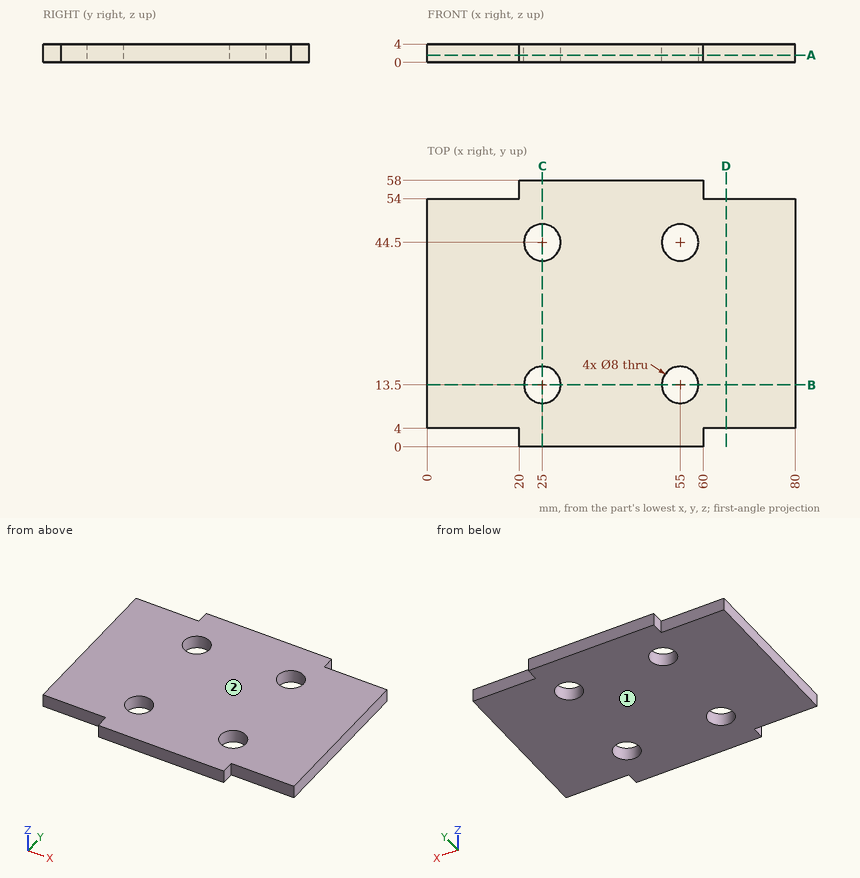
For this review, use the dimensioned drawing (mm, ordinates from the lowest corner) and the shaded views. Give positions to 0.01 mm unless a question says otherwise; leave off trailing zeros. Order: outer loops, then holes, each group sorted by start corner. A loop starts at its lowest first (then second) coordinate and runs counter-clockwise, first axis right, second up. Notation, with made-up numbers: (34, -26) - (87, -26) arc R22 cw to (87, -13) - close; hole circle Ø11 at (59.5, 64). An arc over 180 degrees is marked (long way). Use a Markdown table: item, result. Add a question column.
(1) Add section B-B on y = 13.5. Give the boundary of the cut face in (x, z), then the cut area to 3 significant figures.
(2) Add section D-D on x = 65. Give the boundary of the cut face in (y, z), then the cut area to 3 significant figures.
(3) Add section A-A on z = 1.6. Give the boundary of the cut face in (x, y), then the cut area to 3 significant figures.
(4) Mouldability with a two-part tool opening along Z and no side actions: class the marked faces 1 and 2 as +Z half, -Z half, draft (parallel to the pull), parting line (faces both ways), or undercut.
(5) Clearance check with flat-ended pins moving along their axes: P1, Ø1.2, axis at x = 66, z = 2, coming from the +Y side; P2, Ø5, axis at x = 55, y = 44.5, coming from the +Z side; P3, Ø2, axis at y = 1.5, z = 2.5, coming from the -X side. State where each tip first meets the part, or that it passes through.
(6) Add section C-C on x = 25. Give the boundary of the cut face in (y, z).
(7) Wall thickness on probe 1 along Y at (x, z) = (55, 3.2); probe 2 along X at (y, z) = (14.5, 3.5); probe 3 along Y at (x, z) = (73, 2.7): over which ranges is each line inside the solid? List them lowest first. Write a range as [from, to].
Report:
| question | item | result |
|---|---|---|
| 1 | outline | (0, 0) - (21, 0) - (21, 4) - (0, 4) - close; (29, 0) - (51, 0) - (51, 4) - (29, 4) - close; (59, 0) - (80, 0) - (80, 4) - (59, 4) - close |
| 1 | area | 256 mm² |
| 2 | outline | (4, 0) - (54, 0) - (54, 4) - (4, 4) - close |
| 2 | area | 200 mm² |
| 3 | outline | (0, 4) - (20, 4) - (20, 0) - (60, 0) - (60, 4) - (80, 4) - (80, 54) - (60, 54) - (60, 58) - (20, 58) - (20, 54) - (0, 54) - close; hole circle Ø8 at (25, 13.5); hole circle Ø8 at (25, 44.5); hole circle Ø8 at (55, 13.5); hole circle Ø8 at (55, 44.5) |
| 3 | area | 4,120 mm² |
| 4 | face 1 | -Z half |
| 4 | face 2 | +Z half |
| 5 | P1 | stops at y = 54 |
| 5 | P2 | passes through |
| 5 | P3 | stops at x = 20 |
| 6 | outline | (0, 0) - (9.5, 0) - (9.5, 4) - (0, 4) - close; (17.5, 0) - (40.5, 0) - (40.5, 4) - (17.5, 4) - close; (48.5, 0) - (58, 0) - (58, 4) - (48.5, 4) - close |
| 7 | probe 1 | y = [0, 9.5], [17.5, 40.5], [48.5, 58] |
| 7 | probe 2 | x = [0, 21.13], [28.87, 51.13], [58.87, 80] |
| 7 | probe 3 | y = [4, 54] |
